Verification items for the finished model (mm, model axes). A direction names the side the tool comes from. Coordinates: 2 decimals unless noted, no trailing zeros. Write each loop counter-clockwise with the first axis right and the second up, starting at its lowest first coordinate (ties: lowest second). Pieces come first, ordered by that corner, then holes.
```python
from build123d import *

# Parameters (mm, degrees)
ESQUISSE1_R                  = 7.5
BOSS_EXTRU_1_DEPTH           = 12
ESQUISSE2_R                  = 7.5
ESQUISSE2_R_2                = 6
ENL_V_MAT_EXTRU_1_DEPTH      = 11
ESQUISSE3_R                  = 3
ENL_V_MAT_EXTRU_2_DEPTH      = 5
ESQUISSE4_W                  = 19.769622122
ESQUISSE4_H                  = 8
ENL_V_MAT_EXTRU_3_DEPTH      = 7
ESQUISSE5_R                  = 1
ENL_V_MAT_EXTRU_4_DEPTH      = 7
ENL_V_MAT_EXTRU_4_DEPTH_BACK = 7
CHANFREIN1_SIZE              = 0.5


with BuildPart() as part:
    # Esquisse1 → Boss.-Extru.1 (new body)
    with BuildSketch(Plane.XY):
        Circle(ESQUISSE1_R)
    extrude(amount=BOSS_EXTRU_1_DEPTH)

    # Esquisse2 → Enlèv. mat.-Extru.1 (cut)
    with BuildSketch(Plane.XY.offset(12)):
        Circle(ESQUISSE2_R)
        Circle(ESQUISSE2_R_2, mode=Mode.SUBTRACT)
    extrude(amount=-ENL_V_MAT_EXTRU_1_DEPTH, mode=Mode.SUBTRACT)

    # Esquisse3 → Enlèv. mat.-Extru.2 (cut)
    with BuildSketch(Plane.XY.offset(12)):
        Circle(ESQUISSE3_R)
    extrude(amount=-ENL_V_MAT_EXTRU_2_DEPTH, mode=Mode.SUBTRACT)

    # Esquisse4 → Enlèv. mat.-Extru.3 (cut)
    with BuildSketch(Plane(origin=(0, 0, 0), x_dir=(-1, 0, 0), z_dir=(0, 0, -1))):
        Rectangle(ESQUISSE4_W, ESQUISSE4_H)
    extrude(amount=-ENL_V_MAT_EXTRU_3_DEPTH, mode=Mode.SUBTRACT)

    # Esquisse5 → Enlèv. mat.-Extru.4 (cut, two sides)
    with BuildSketch(Plane(origin=(0, 0, 0), x_dir=(1, 0, 0), z_dir=(0, 1, 0))) as enl_v_mat_extru_4_sk:
        with Locations((0, -9)):
            Circle(ESQUISSE5_R)
    extrude(amount=ENL_V_MAT_EXTRU_4_DEPTH, mode=Mode.SUBTRACT)
    extrude(enl_v_mat_extru_4_sk.sketch, amount=-ENL_V_MAT_EXTRU_4_DEPTH_BACK, mode=Mode.SUBTRACT)

    # Chanfrein1
    chanfrein1_edges = [part.edges().sort_by_distance(p)[0] for p in [
        (-6, 0, 12),
    ]]
    chamfer(chanfrein1_edges, length=CHANFREIN1_SIZE)


solid = part.part
```
1. Sectioned sample at B-B, the plane x = 0. Record the boundary of the cut face in (y, z), and give its area (4 significant figures).
2. Material ranges on L1, parallel to Z at x = 0, y = 3.7; L2, parallel to Z at x = 0, y = 4.2; L3, parallel to Z at x = 4, y = -1.5, recorded low to high.
3. Draft check along Y on faces 1 (the cylindrical face through (1, -4, 9)), 2 (the cylindrical face through (-0.1, -7.5, 0.5)), 3 (the flat face through (0, -4, 3)). Enter one of: pulls with the +Y half, pulls with the -Y half, needs draft (parallel to the pull), parting line crosses it, or undercut.
4. Gauge pin test, flat ends, axial feed: P1, Ø2, axis at x = -1.5, z = 8, coming from the -Y side; P2, Ø1.1, axis at x = 0, y = -6.5, coming from the +Z side; P3, Ø3.5, axis at x = 0, z = 5, coming from the +Y side. Record the tip position at first contact, or that the pin passes through.
5. Sectioned sample at A-A, the plane y = 0. Record the boundary of the cut face in (x, z), and give its area (4 significant figures).
6. Sectioned sample at D-D, the plane z = 2.25. Record the boundary of the cut face in (x, y).
7. Tool access check on faces 4 (the flat face through (-3, 2, 7)), 5 (the cylindrical face through (-0.78, 5.95, 7.49)), 6 (the flat face through (0, -7, 1)). Record the directions out of +Z, -Z, +X, -X, +Y, -Y that give a thin tool (end or side, any length) a straight path to the whole face; none if there is none.
8. Sectioned sample at C-C, the plane z = 8.5. Record the boundary of the cut face in (x, y).
Outcome:
1. outline: (-7.5, 0) - (-4, 0) - (-4, 7) - (-3, 7) - (-3, 8) - (-6, 8) - (-6, 1) - (-7.5, 1) - close; (-6, 10) - (-3, 10) - (-3, 12) - (-5.5, 12) - (-6, 11.5) - close; (3, 7) - (4, 7) - (4, 0) - (7.5, 0) - (7.5, 1) - (6, 1) - (6, 8) - (3, 8) - close; (3, 10) - (6, 10) - (6, 11.5) - (5.5, 12) - (3, 12) - close
1. area: 48.75 mm2
2. L1: z = 7 to 8, 10 to 12
2. L2: z = 0 to 8, 10 to 12
2. L3: z = 7 to 12
3. face 1: needs draft
3. face 2: pulls with the -Y half
3. face 3: undercut
4. P1: stops at y = -5.98
4. P2: stops at z = 11.55
4. P3: stops at y = 6
5. outline: (-6, 7) - (-3, 7) - (-3, 12) - (-5.5, 12) - (-6, 11.5) - close; (3, 7) - (6, 7) - (6, 11.5) - (5.5, 12) - (3, 12) - close
5. area: 29.75 mm2
6. outline: (-4.47, -4) arc R6 ccw to (4.47, -4) - close; (-4.47, 4) - (4.47, 4) arc R6 ccw to start
7. face 4: -Z, +X, -X
7. face 5: +Z
7. face 6: +Z, -Y
8. outline: (-0.87, -5.94) - (-0.87, -2.87) arc R3 cw to (-0.87, 2.87) - (-0.87, 5.94) arc R6 ccw to start; (0.87, -5.94) arc R6 ccw to (0.87, 5.94) - (0.87, 2.87) arc R3 cw to (0.87, -2.87) - close
